Check sheet for the modelled part. Datum: model origin and axes. Units: mm. Give positions to 0.01 mm unless a question says otherwise; leave off trailing zeros. Loops run counter-clockwise (first coordinate to the right, second up) from the corner with the lowest first, then second, coordinate; pieces in that order, holes last. Notation, with made-up numbers: (36, -17.75) - (72, -17.75) arc R23 ccw to (72, -7.75) - close; hole circle Ø11 at (-28.75, -33). An arc over 180 degrees is marked (long way). Answer in a Markdown table with one row per item. Add a question column.
(1) Sectioned sample at C-C on z = 39. Enter the section's corners in (x, y), then the cut area to 3 significant figures.
(2) Thickness scan on L1, parallel to Z at x = 0, y = -1; L2, parallel to Z at x = -6, y = -15; L3, parallel to X at y = 3, z = 36. Record the ranges inside material, lowest first.
(3) Sectioned sample at B-B on z = 20. Enter the section's corners in (x, y), then the cut area to 3 significant figures.
(4) Go/stop test with flat-tipped pins: P1, Ø8, axis at y = -7.5, z = 8, coming from the -X side; P2, Ø6, axis at x = -12.5, z = 48.5, coming from the +Y side; P3, Ø6, axis at x = 8.5, z = 50.5, coming from the +Y side. Record where each tip stops, or that it passes through.
(5) Sectioned sample at A-A on z = 28. Enter the section's corners in (x, y).
from build123d import *

# Parameters (mm, degrees)
F4_DEPTH       = 21.5910001
F5_DEPTH       = 21.5910001
F6_DEPTH       = 21.5910001
F7_DEPTH       = 21.5910001
F8_DEPTH       = 21.5910001
F9_DEPTH       = 21.5910001
F11_DEPTH      = 21.5910001
F12_DEPTH      = 21.5910001
F12_DEPTH_BACK = 25.4


with BuildPart() as f1:
    # F0 (on Front) → F1 (revolve)
    with BuildSketch(Plane.XZ):
        with BuildLine():
            Line((-21.59, 0), (0, 0))
            Line((0, 0), (0, 66.294))
            ThreePointArc((0, 66.294), (-11.7291440927, 63.9276179966), (-21.59, 57.15))
            Line((-21.59, 57.15), (-21.59, 0))
        make_face()
    revolve(axis=Axis((0, 0, 33.147), (0, 0, 1)))

    # F3 (on Front) → F4 (cut, through all)
    with BuildSketch(Plane.XZ):
        with BuildLine():
            ThreePointArc((0, 25.146), (6.9147972132, 28.0102027868), (9.779, 34.925))
            ThreePointArc((9.779, 34.925), (-6.9147972132, 41.8397972132), (0, 25.146))
        make_face()
    extrude(amount=-F4_DEPTH, mode=Mode.SUBTRACT)

    # F2 (on Front) → F5 (cut, through all)
    with BuildSketch(Plane.XZ):
        with BuildLine():
            ThreePointArc((0, 25.146), (6.9147972132, 28.0102027868), (9.779, 34.925))
            ThreePointArc((9.779, 34.925), (-6.9147972132, 41.8397972132), (0, 25.146))
        make_face()
    extrude(amount=-F5_DEPTH, mode=Mode.SUBTRACT)

    # F3 (on Front) → F6 (cut, through all)
    with BuildSketch(Plane.XZ):
        with BuildLine():
            ThreePointArc((0, 25.146), (6.9147972132, 28.0102027868), (9.779, 34.925))
            ThreePointArc((9.779, 34.925), (-6.9147972132, 41.8397972132), (0, 25.146))
        make_face()
    extrude(amount=-F6_DEPTH, mode=Mode.SUBTRACT)

    # F3 (on Front) → F7 (cut, through all)
    with BuildSketch(Plane.XZ):
        with BuildLine():
            ThreePointArc((0, 25.146), (6.9147972132, 28.0102027868), (9.779, 34.925))
            ThreePointArc((9.779, 34.925), (-6.9147972132, 41.8397972132), (0, 25.146))
        make_face()
    extrude(amount=-F7_DEPTH, mode=Mode.SUBTRACT)

    # F3 (on Front) → F8 (cut, through all)
    with BuildSketch(Plane.XZ):
        with BuildLine():
            ThreePointArc((0, 25.146), (6.9147972132, 28.0102027868), (9.779, 34.925))
            ThreePointArc((9.779, 34.925), (-6.9147972132, 41.8397972132), (0, 25.146))
        make_face()
    extrude(amount=-F8_DEPTH, mode=Mode.SUBTRACT)

    # F3 (on Front) → F9 (cut, through all)
    with BuildSketch(Plane.XZ):
        with BuildLine():
            ThreePointArc((0, 25.146), (6.9147972132, 28.0102027868), (9.779, 34.925))
            ThreePointArc((9.779, 34.925), (-6.9147972132, 41.8397972132), (0, 25.146))
        make_face()
    extrude(amount=-F9_DEPTH, mode=Mode.SUBTRACT)

    # F3 (on Front) → F11 (cut, through all)
    with BuildSketch(Plane.XZ):
        with BuildLine():
            ThreePointArc((0, 25.146), (6.9147972132, 28.0102027868), (9.779, 34.925))
            ThreePointArc((9.779, 34.925), (-6.9147972132, 41.8397972132), (0, 25.146))
        make_face()
    extrude(amount=-F11_DEPTH, mode=Mode.SUBTRACT)

    # F10 (on Front) → F12 (cut, two sides)
    with BuildSketch(Plane.XZ) as f12_sk:
        with BuildLine():
            ThreePointArc((0, 25.3496200125), (6.9147972132, 28.2138227993), (9.779, 35.1286200125))
            ThreePointArc((9.779, 35.1286200125), (-6.9147972132, 42.0434172257), (0, 25.3496200125))
        make_face()
    extrude(amount=-F12_DEPTH, mode=Mode.SUBTRACT)
    extrude(f12_sk.sketch, amount=F12_DEPTH_BACK, mode=Mode.SUBTRACT)


solid = f1.part
Reply:
| question | item | result |
|---|---|---|
| 1 | outline | (-8.98, -19.63) - (-8.98, 19.63) arc R21.59 ccw to start; (8.98, -19.63) arc R21.59 ccw to (8.98, 19.63) - close |
| 1 | area | 712 mm^2 |
| 2 | L1 | 0 to 25.35, 44.91 to 66.28 |
| 2 | L2 | 0 to 27.41, 42.85 to 61.6 |
| 2 | L3 | -21.38 to -9.74, 9.74 to 21.38 |
| 3 | outline | circle Ø43.18 at (0, 0) |
| 3 | area | 1,460 mm^2 |
| 4 | P1 | x = -21.3 |
| 4 | P2 | y = 19.39 |
| 4 | P3 | y = 20.88 |
| 5 | outline | (-6.9, 0) - (-6.9, 20.46) arc R21.59 ccw to (-6.69, -20.53) - (-6.69, 0) - close; (6.69, -20.53) arc R21.59 ccw to (6.9, 20.46) - (6.9, 0) - (6.69, 0) - close |
